```python
from build123d import *

# Parameters (mm, degrees)
SKETCH1_R               = 4.953
BOSS_EXTRUDE1_DEPTH     = 25.4
SKETCH2_R               = 6.858
BOSS_EXTRUDE2_DEPTH     = 2.032
CUT_EXTRUDE1_DEPTH      = 28.188680145
CUT_EXTRUDE1_DEPTH_BACK = 28.188680145
SKETCH3_W               = 1.27
SKETCH3_H               = 2.794


with BuildPart() as part:
    # Sketch1 → Boss-Extrude1 (new body)
    with BuildSketch(Plane.XY):
        Circle(SKETCH1_R)
    extrude(amount=BOSS_EXTRUDE1_DEPTH)

    # Sketch2 → Boss-Extrude2 (add)
    with BuildSketch(Plane.XY.offset(25.4)):
        Circle(SKETCH2_R)
    extrude(amount=-BOSS_EXTRUDE2_DEPTH)

    # Sketch3 → Cut-Extrude1 (cut, two sides: drawn at the far end of the back side and taken through both)
    with BuildSketch(Plane(origin=(0, 0, 0), x_dir=(1, 0, 0), z_dir=(0, 1, 0)).offset(-CUT_EXTRUDE1_DEPTH_BACK)):
        with Locations((4.318, -2.667)):
            Rectangle(SKETCH3_W, SKETCH3_H)
        with Locations((-4.318, -2.667)):
            Rectangle(SKETCH3_W, SKETCH3_H)
    extrude(amount=CUT_EXTRUDE1_DEPTH + CUT_EXTRUDE1_DEPTH_BACK, mode=Mode.SUBTRACT)


solid = part.part
```
Part model, mm, in its own coordinate system. A direction names the side the tool comes from. Give positions to 0.01 mm unless a question says otherwise; leave off trailing zeros. Loops run counter-clockwise (first coordinate to the right, second up) from the corner with the lowest first, then second, coordinate; pieces in that order, holes last. Notation, with made-up numbers: M -26,50.5 L -12,50.5 A25 cw -12,71.5 Z; hole C 89.5,3 d11. An arc over 180 degrees is marked long. Return JSON: item names as keys, results as strings.
1) Drill centre lines: line 1 (Z direction, x = -2.75, y = 5.5); line 2 (X direction, y = 0, z = 9.75). Where is each one in solid material? Low to high.
Calculated:
{"line 1": "z = 23.37 to 25.4", "line 2": "x = -4.95 to 4.95"}
2) Saw through at D-D, the plane y = 1.75. List the corners of the cut face in (x, z).
Calculated:
{"outline": "M -6.63,23.37 L -4.63,23.37 L -4.63,4.06 L -3.68,4.06 L -3.68,1.27 L -4.63,1.27 L -4.63,0 L 4.63,0 L 4.63,1.27 L 3.68,1.27 L 3.68,4.06 L 4.63,4.06 L 4.63,23.37 L 6.63,23.37 L 6.63,25.4 L -6.63,25.4 Z"}
3) Saw through at B-B, the plane y = 0. List the corners of the cut face in (x, z).
Calculated:
{"outline": "M -6.86,23.37 L -4.95,23.37 L -4.95,4.06 L -3.68,4.06 L -3.68,1.27 L -4.95,1.27 L -4.95,0 L 4.95,0 L 4.95,1.27 L 3.68,1.27 L 3.68,4.06 L 4.95,4.06 L 4.95,23.37 L 6.86,23.37 L 6.86,25.4 L -6.86,25.4 Z"}
4) Pull direction Z, two halves, no side cores. Call faces 1 (the face through (3.683, 0, 3)), 2 (the face through (-1.487, -6.695, 24.398)), 3 (the face through (0, 0, 0)): released by +Z, released by -Z, zero draft, split by the parting line, or undercut.
Calculated:
{"face 1": "undercut", "face 2": "zero draft", "face 3": "released by -Z"}
5) Flat gauge pins, fed straight in: pin 1 Ø3 at (y, z) = (0, 2) entering from +X; pin 2 Ø2 at (y, z) = (5, 19) entering from +X; pin 3 Ø4 at (x, z) = (-2.5, 11) entering from +Y. Where does each tip first touch, or does it go through?
Calculated:
{"pin 1": "stops at x = 4.95", "pin 2": "stops at x = 2.92", "pin 3": "stops at y = 4.93"}
6) 3-axis set-ups, long thin cutter, end or side, ignore diameter. For faces 4 (the face through (-3.683, 0, 3)), 5 (the face through (0, 0, 25.4)), 6 (the face through (4, 0, 1.27)), 7 (the face through (2, -5, 23.368)): which of +Z, -Z, +X, -X, +Y, -Y reach the whole face in a straight line?
Calculated:
{"face 4": "-X, +Y, -Y", "face 5": "+Z, +X, -X, +Y, -Y", "face 6": "+X, +Y, -Y", "face 7": "-Z"}
7) Saw through at C-C, the plane z = 7.5. List the corners of the cut face in (x, y).
Calculated:
{"outline": "C 0,0 d9.91"}
8) Saw through at A-A, the plane x = 0. List the corners of the cut face in (y, z), then the cut area to 3 significant figures.
Calculated:
{"outline": "M -6.86,23.37 L -4.95,23.37 L -4.95,0 L 4.95,0 L 4.95,23.37 L 6.86,23.37 L 6.86,25.4 L -6.86,25.4 Z", "area": "259 mm2"}
